Autodesk Inventor part; units mm, degrees
ref_plane "YZ Plane" through (0, 0, 0) normal (1, 0, 0) x (0, 1, 0)
ref_plane "XZ Plane" through (0, 0, 0) normal (0, 1, 0) x (-1, 0, 0)
ref_plane "XY Plane" through (0, 0, 0) normal (0, 0, 1) x (1, 0, 0)
sketch "Эскиз1" plane through (0, 0, 0) normal (0, 0, 1) x (1, 0, 0)
  circle A0 centre (0, 0) radius 13.8038
  circle A1 centre (0, 0) radius 9.815
  line L0 (-3.05, 2.51) -> (-3.05, 9.3291)
  line L1 (3.05, 9.3291) -> (3.05, 2.51)
  line L2 (-3.05, -9.3291) -> (-3.05, -2.51)
  line L3 (3.05, -2.51) -> (3.05, -9.3291)
  line L4 (-3.05, -2.51) -> (-3.05, 2.51)
  line L5 (3.05, -2.51) -> (3.05, 2.51)
  circle A2 centre (0, 0) radius 10.1941
extrude "Выдавливание1" add sketch "Эскиз1" along normal blind 3 contours A0
sketch "Эскиз2" plane through (0, 0, 0) normal (0, 0, -1) x (-1, 0, 0)
  line L0 (-3.05, 9.3291) -> (-3.05, 2.51)
  circle A0 centre (0, 0) radius 3.95
  line L1 (-3.05, -2.51) -> (-3.05, -9.3291)
  line L2 (3.05, -9.3291) -> (3.05, -2.51)
  line L3 (3.05, 2.51) -> (3.05, 9.3291)
  line L4 (-3.05, -9.3291) -> (-3.05, -9.7271)
  circle A1 centre (0, 0) radius 10.1941
  line L5 (3.05, -9.3291) -> (3.05, -9.7271)
  line L6 (-3.05, 9.3291) -> (-3.05, 9.7271)
  line L7 (3.05, 9.3291) -> (3.05, 9.7271)
extrude "Выдавливание2" add sketch "Эскиз2" against normal blind 1 contours L0 A0 L1 L4 A1 L6 | L3 L7 A1 L5 L2 A0
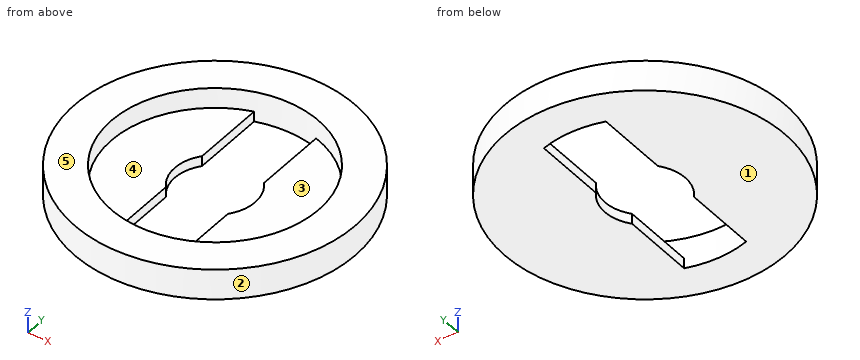
Can you work these out from the model? Positions are in its coordinate system, mm. Face numbers are marked on the shaded views. A direction names the side the tool comes from. Coordinates: 2 decimals unless noted, no trailing zeros. Loops run counter-clockwise (first coordinate to the right, second up) from the corner with the lowest first, then second, coordinate; pieces in that order, holes last. Notation, with made-up numbers: (-25.5, 34.5) -> (25.5, 34.5) arc R21 cw to (25.5, 43.5) -> close; hole circle Ø3 at (47, 7). An arc over 180 degrees is marked (long way). Put each result on its own line as item: value. Start each with the question number.
Q1. For the marked faces 4 and 5, which set-ups out of +Z, -Z, +X, -X, +Y, -Y let a thin tool reach every point of the face, with its end or its side?
Q2. I want a section at A-A (x = 0). Write out the boundary of the cut face in (y, z).
Q3. I want a section at B-B (y = 0). Write out the boundary of the cut face in (x, z), plus the area to 3 significant figures.
Q4. I want a section at D-D (x = -4.75). Write out the boundary of the cut face in (y, z), plus the area to 3 significant figures.
Q5. If I drill on line 1 (Y direction, x = 0, z = 2.15); line 2 (X direction, y = 8.25, z = 0.75); line 3 (X direction, y = 5.75, z = 1.55), over which ranges is the centre line in solid material (lowest first)? Write a range as [from, to].
Q6. Thinking about a two-plate mould opening in X: for the marked faces 1, 2 and 3, which applies, pulls with the +X half, pulls with the -X half, needs draft (parallel to the pull), parting line crosses it, or undercut?
Q7. I'm going to push flat-ended pins straight in: P1, Ø0.8, axis at y = -4.5, z = 0.5, coming from the -X side; P2, Ø0.8, axis at y = 8, z = 0.5, coming from the +X side; P3, Ø3, axis at x = 1.5, y = -1, coming from the +Z side; P4, Ø2, axis at x = 3.5, y = 1.5, coming from the +Z side. Where does each tip first touch, or does it pass through?
Q8. I want a section at C-C (z = 2.4). Write out the boundary of the cut face in (x, y).
Taken from the geometry:
1. face 4: +Z
1. face 5: +Z, +X, -X, +Y, -Y
2. outline: (-13.8, 0) -> (-10.19, 0) -> (-10.19, 3) -> (-13.8, 3) -> close; (10.19, 0) -> (13.8, 0) -> (13.8, 3) -> (10.19, 3) -> close
3. outline: (-13.8, 0) -> (-3.95, 0) -> (-3.95, 1) -> (-10.19, 1) -> (-10.19, 3) -> (-13.8, 3) -> close; (3.95, 0) -> (13.8, 0) -> (13.8, 3) -> (10.19, 3) -> (10.19, 1) -> (3.95, 1) -> close
3. area: 34.1 mm2
4. outline: (-12.96, 0) -> (12.96, 0) -> (12.96, 3) -> (9.02, 3) -> (9.02, 1) -> (-9.02, 1) -> (-9.02, 3) -> (-12.96, 3) -> close
4. area: 41.7 mm2
5. line 1: y = [-13.8, -10.19], [10.19, 13.8]
5. line 2: x = [-11.07, -3.05], [3.05, 11.07]
5. line 3: x = [-12.55, -8.42], [8.42, 12.55]
6. face 1: needs draft
6. face 2: parting line crosses it
6. face 3: undercut
7. P1: stops at x = -13.18
7. P2: stops at x = 11.52
7. P3: passes through
7. P4: stops at z = 1
8. outline: circle Ø27.61 at (0, 0); hole circle Ø20.39 at (0, 0)
